Source: three-view drawing plus pictorial views. Frame: mm from the lowest corner of the part. A direction names the side the tool comes from. Give positions to 0.01 mm unless a question says otherwise; leave off trailing zeros. Write each loop counter-clockwise with the first axis right and the second up, starting at its lowest first coordinate (ties: lowest second). Pieces come first, ordered by that corner, then holes. Notation, with made-up numbers: M 50.25,-18.5 L 74.25,-18.5 A32 ccw 74.25,14.5 Z; hole C 86.25,51 d4. An arc over 180 degrees is marked long. Return JSON: item names as keys, results as strings.
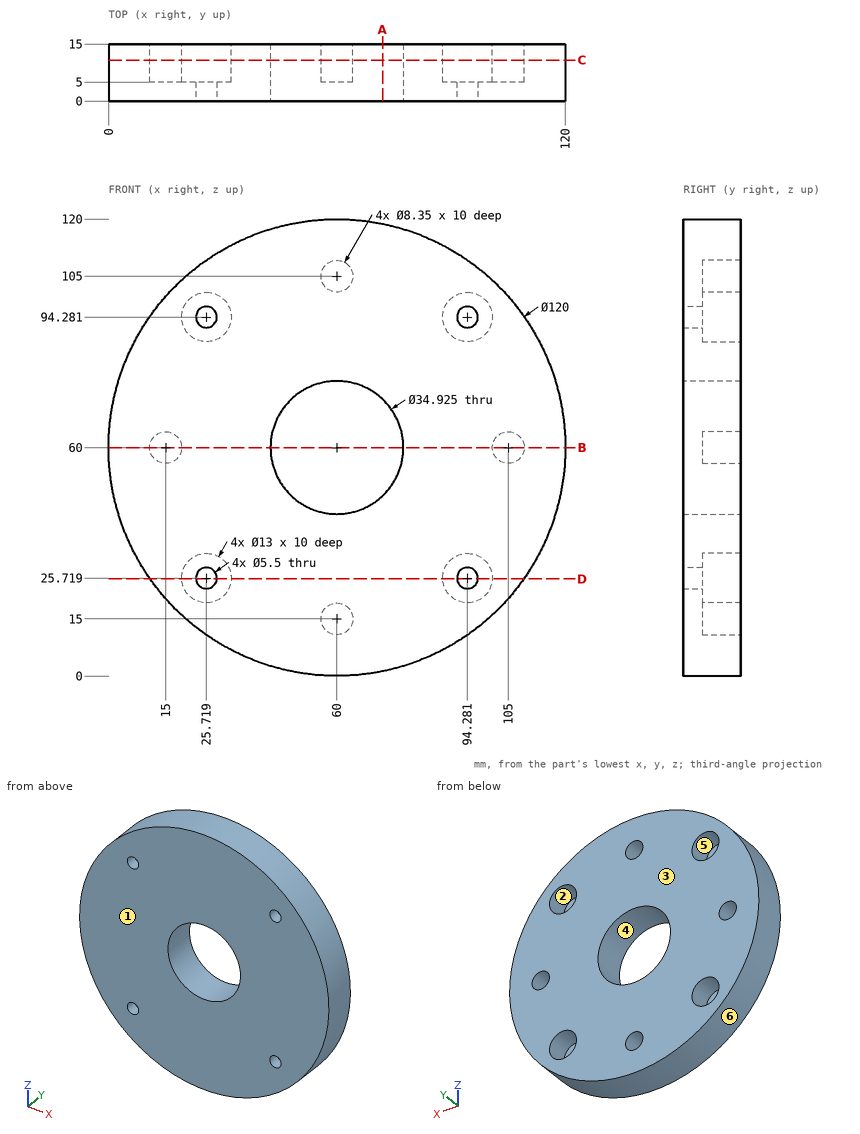
1) Cut plane D-D, the plane z = 25.5. Return the cut outline in (x, y) (1 decimal).
Numbers:
{"outline": "M 10.9,0 L 23,0 L 23,5 L 19.2,5 L 19.2,15 L 10.9,15 Z; M 28.5,0 L 91.5,0 L 91.5,5 L 87.8,5 L 87.8,15 L 32.2,15 L 32.2,5 L 28.5,5 Z; M 97,0 L 109.1,0 L 109.1,15 L 100.8,15 L 100.8,5 L 97,5 Z"}
2) Cut plane A-A, the plane x = 72. Return the cut outline in (y, z).
Numbers:
{"outline": "M 0,1.21 L 15,1.21 L 15,47.31 L 0,47.31 Z; M 0,72.69 L 15,72.69 L 15,118.79 L 0,118.79 Z"}
3) Line query: line 1 (Z direction, x = 60.5, y = 9.5) (1 decimal); line 2 (X direction, y = 14, z = 95) (1 decimal); line 3 (Z direction, x = 58, y = 10.5) (1 decimal). Output: solid intervals per line, ascending. Write a range as [from, to].
Numbers:
{"line 1": "z = [0, 10.9], [19.1, 42.5], [77.5, 100.9], [109.1, 120]", "line 2": "x = [11.3, 19.3], [32.2, 87.8], [100.7, 108.7]", "line 3": "z = [0, 11.3], [18.7, 42.7], [77.3, 101.3], [108.7, 120]"}
4) Draft query along X for the marked faces 3, 4, 5 and 6. Return one class per face: released by +X, released by -X, zero draft, split by the parting line, or undercut.
Numbers:
{"face 3": "zero draft", "face 4": "undercut", "face 5": "undercut", "face 6": "split by the parting line"}
5) Set-up query: the marked faces 1 and 2. Return all of +Z, -Z, +X, -X, +Y, -Y with unobstructed straight access to the full face (end or side cutting, diameter ignored); none if empty.
Numbers:
{"face 1": "+Z, -Z, +X, -X, -Y", "face 2": "+Y"}
6) Contact query for flat-ended pins moving along their axis: pin 1 Ø4 at (x, z) = (25.5, 94) entering from +Y; pin 2 Ø1.5 at (x, y) = (68, 9.5) entering from -Z; pin 3 Ø6 at (x, y) = (32, 10) entering from +Z; pin 4 Ø4 at (x, y) = (62.5, 13) entering from -Z. Output: stop coordinate, or through.
Numbers:
{"pin 1": "passes through", "pin 2": "stops at z = 0.44", "pin 3": "stops at z = 114.54", "pin 4": "stops at z = 0"}
7) Cut plane B-B, the plane z = 60. Return the cut outline in (x, y) (1 decimal).
Numbers:
{"outline": "M 0,0 L 42.5,0 L 42.5,15 L 19.2,15 L 19.2,5 L 10.8,5 L 10.8,15 L 0,15 Z; M 77.5,0 L 120,0 L 120,15 L 109.2,15 L 109.2,5 L 100.8,5 L 100.8,15 L 77.5,15 Z"}
8) Cut plane C-C, the plane y = 10.75. Give the number of separate pieces and of enclosed holes in the cut face, then the cut area to 3 significant figures.
Numbers:
{"separate pieces": "1", "enclosed holes": "9", "area": "9,600 mm²"}
